Geometry check sheet. Reference: the model listing, model coordinates, mm. Face numbers are marked on the shaded views. A direction names the side the tool comes from. Give positions to 0.01 mm unless a question says otherwise; leave off trailing zeros. Write each loop counter-clockwise with the first axis right and the second up, starting at its lowest first coordinate (ties: lowest second). Pieces come first, ordered by that corner, then holes. Notation, with made-up numbers: (69, -14.75) -> (90, -14.75) arc R34 ccw to (90, 24.25) -> close; hole circle Ø3 at (62, 10). An arc over 180 degrees is marked (long way). Write item = value, one per line. Start each with the question number.
1. Thickness scan on line 1 along Z through (x, y) = (1, -2.5); line 2 along Z through (x, y) = (1.25, -9.5); line 3 along X through (y, z) = (-10.75, 3.75). Record the ranges inside material, lowest first.
2. Cross-section at C-C, the plane y = -3.25. Record the cut outline in (x, z), plus the area to 3 significant figures.
3. Cross-section at B-B, the plane x = 2.25. Record the cut outline in (y, z).
4. Cross-section at D-D, the plane z = 3.25. Record the cut outline in (x, y), plus the area to 3 significant figures.
5. Depth check by flat-ended pin: P1, Ø2, axis at x = 6, z = -2, coming from the -Y side; P2, Ø3.5, axis at y = -5.5, z = 1, coming from the +X side; P3, Ø3, axis at x = 6, y = -5, coming from the +Z side. Enter the tip coordinate at first touch or a pass-through.
6. Cross-section at A-A, the plane y = -8.75. Record the cut outline in (x, z).
7. Mould release check, pull along Y, two halves, no side actions. Record for the marked faces 1, 2 and 3: pulls with the +Y half, pulls with the -Y half, needs draft (parallel to the pull), parting line crosses it, or undercut.
8. Set-up check for the marked faces 4 and 5: record each of +Z, -Z, +X, -X, +Y, -Y from which the full face is reachable in a straight line by a thin tool's end or side.
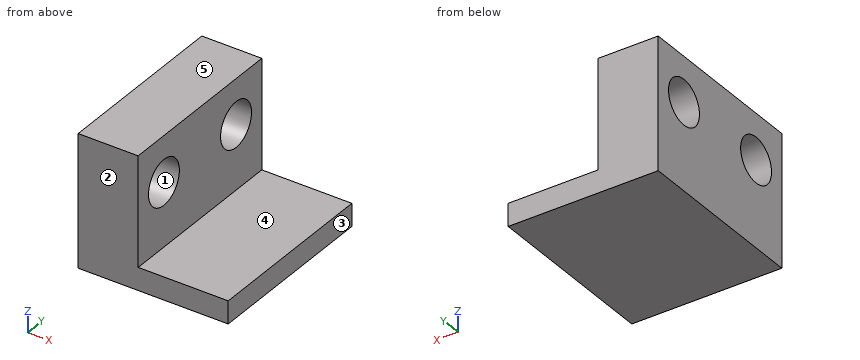
```python
from build123d import *

# Parameters (mm, degrees)
F0_W     = 6
F0_H     = 1.511796
F1_DEPTH = 12
F2_R     = 1.5
F3_DEPTH = 25


with BuildPart() as f1:
    # F0 (on Front) → F1 (new body)
    with BuildSketch(Plane.XZ):
        with Locations((5, -3.644102)):
            Rectangle(F0_W, F0_H)
        Polygon((-2, -4.4), (2, -4.4), (2, -2.888204), (2, 4.4), (-2, 4.4), align=None)
    extrude(amount=F1_DEPTH)

    # F2 (on face) → F3 (cut)
    with BuildSketch(Plane(origin=(-2, 0, 0), x_dir=(0, -1, 0), z_dir=(-1, 0, 0))):
        with Locations((2.5, 1.4)):
            Circle(F2_R)
        with Locations((9.499757, 1.341669)):
            Circle(F2_R)
    extrude(amount=-F3_DEPTH, mode=Mode.SUBTRACT)


solid = f1.part
```
Answers:
q1.line_1 = -4.4 to -0.1, 2.9 to 4.4
q1.line_2 = -4.4 to -0.16, 2.84 to 4.4
q1.line_3 = -2 to 2
q2.outline = (-2, -4.4) -> (8, -4.4) -> (8, -2.89) -> (2, -2.89) -> (2, 0.1) -> (-2, 0.1) -> close; (-2, 2.7) -> (2, 2.7) -> (2, 4.4) -> (-2, 4.4) -> close
q2.area = 33.9 mm^2
q3.outline = (-12, -4.4) -> (0, -4.4) -> (0, -2.89) -> (-12, -2.89) -> close
q4.outline = (-2, -12) -> (2, -12) -> (2, 0) -> (-2, 0) -> close
q4.area = 48.0 mm^2
q5.P1 = -12
q5.P2 = 2
q5.P3 = -2.89
q6.outline = (-2, -4.4) -> (8, -4.4) -> (8, -2.89) -> (2, -2.89) -> (2, 0.04) -> (-2, 0.04) -> close; (-2, 2.64) -> (2, 2.64) -> (2, 4.4) -> (-2, 4.4) -> close
q7.face_1 = undercut
q7.face_2 = pulls with the -Y half
q7.face_3 = needs draft
q8.face_4 = +Z, +X, +Y, -Y
q8.face_5 = +Z, +X, -X, +Y, -Y
